Verification items for the finished model (mm, model axes). A direction names the side the tool comes from. Give positions to 0.01 mm unless a question says otherwise; leave off trailing zeros. Write each loop counter-clockwise with the first axis right and the second up, starting at its lowest first coordinate (ties: lowest second). Pieces come first, ordered by that corner, then holes. Notation, with made-up numbers: (-34, 77) -> (-16, 77) arc R18 ccw to (-16, 96) -> close; hole circle Ø9 at (-13.75, 32.5). An arc over 180 degrees is marked (long way). Write item = value, one per line.
from build123d import *

# Parameters (mm, degrees)
F0_R     = 4.5
F0_R_2   = 1.5
F1_DEPTH = 1.5
F2_R     = 4


with BuildPart() as f1:
    # F0 (on Top) → F1 (new body)
    with BuildSketch(Plane.XY):
        with BuildLine():
            ThreePointArc((3.004161691, -5.7955113904), (1.5522577141, -6.3433300134), (0.0118794416, -6.5313863328))
            ThreePointArc((0.0118794416, -6.5313863328), (-1.5361614481, -6.3472667251), (-2.995838309, -5.7998417643))
            Line((-2.995838309, -5.7998417643), (-2.995838309, -10.8488196837))
            ThreePointArc((-2.995838309, -10.8488196837), (-2.764421371, -11.4885696949), (-2.1772781553, -11.8322217287))
            ThreePointArc((-2.1772781553, -11.8322217287), (0.0046169816, -12.0313963001), (2.1863582083, -11.8305428262))
            ThreePointArc((2.1863582083, -11.8305428262), (2.7729908389, -11.4867349425), (3.004161691, -10.8472806897))
            Line((3.004161691, -10.8472806897), (3.004161691, -5.7955113904))
        make_face()
        with BuildLine():
            ThreePointArc((0.0118794416, -6.5313863328), (1.0743113125, -6.9697548816), (1.5146208008, -8.0313838278))
            ThreePointArc((1.5146208008, -8.0313838278), (-1.0450697109, -9.093012774), (0.0118794416, -6.5313863328))
        make_face(mode=Mode.SUBTRACT)
        with BuildLine():
            ThreePointArc((-2.995838309, -5.7998417643), (-1.5361614481, -6.3472667251), (0.0118794416, -6.5313863328))
            ThreePointArc((0.0118794416, -6.5313863328), (1.5522577141, -6.3433300134), (3.004161691, -5.7955113904))
            ThreePointArc((3.004161691, -5.7955113904), (4.5961940777, -4.627591266), (5.7641142021, -3.0355588793))
            ThreePointArc((5.7641142021, -3.0355588793), (6.3133486484, -1.5778863875), (6.5, -0.0313971883))
            ThreePointArc((6.5, -0.0313971883), (6.3144631499, 1.5105350826), (5.768444576, 2.9644411207))
            ThreePointArc((5.768444576, 2.9644411207), (4.5995100863, 4.5614784867), (3.004161691, 5.7327170138))
            ThreePointArc((3.004161691, 5.7327170138), (1.5481312977, 6.2815489928), (0.0033814005, 6.4686019322))
            ThreePointArc((0.0033814005, 6.4686019322), (-1.540289778, 6.2834668165), (-2.995838309, 5.7370473877))
            ThreePointArc((-2.995838309, 5.7370473877), (-4.5961940777, 4.5647968894), (-5.768444576, 2.9644411207))
            ThreePointArc((-5.768444576, 2.9644411207), (-6.4999983071, -0.0360884255), (-5.7641142021, -3.0355588793))
            ThreePointArc((-5.7641142021, -3.0355588793), (-4.592875675, -4.6309072746), (-2.995838309, -5.7998417643))
        make_face()
        with Locations((0, -0.0313971883)):
            Circle(F0_R, mode=Mode.SUBTRACT)
        with BuildLine():
            Line((-10.8158835014, -3.0355588793), (-5.7641142021, -3.0355588793))
            ThreePointArc((-5.7641142021, -3.0355588793), (-6.4999983071, -0.0360884255), (-5.768444576, 2.9644411207))
            Line((-5.768444576, 2.9644411207), (-10.8174224954, 2.9644411207))
            ThreePointArc((-10.8174224954, 2.9644411207), (-11.4571725066, 2.7330241827), (-11.8008245404, 2.145880967))
            ThreePointArc((-11.8008245404, 2.145880967), (-11.9999991118, -0.0360141699), (-11.7991456379, -2.2177553966))
            ThreePointArc((-11.7991456379, -2.2177553966), (-11.4553377541, -2.8043880272), (-10.8158835014, -3.0355588793))
        make_face()
        with Locations((-9.5, -0.0313971883)):
            Circle(F0_R_2, mode=Mode.SUBTRACT)
        with BuildLine():
            ThreePointArc((6.5, -0.0313971883), (6.3133486484, -1.5778863875), (5.7641142021, -3.0355588793))
            Line((5.7641142021, -3.0355588793), (10.8158835014, -3.0355588793))
            ThreePointArc((10.8158835014, -3.0355588793), (11.4553377541, -2.8043880272), (11.7991456379, -2.2177553966))
            ThreePointArc((11.7991456379, -2.2177553966), (11.9999991118, -0.0360141699), (11.8008245404, 2.145880967))
            ThreePointArc((11.8008245404, 2.145880967), (11.4571725066, 2.7330241827), (10.8174224954, 2.9644411207))
            Line((10.8174224954, 2.9644411207), (5.768444576, 2.9644411207))
            ThreePointArc((5.768444576, 2.9644411207), (6.3144631499, 1.5105350826), (6.5, -0.0313971883))
        make_face()
        with Locations((9.5, -0.0313971883)):
            Circle(F0_R_2, mode=Mode.SUBTRACT)
        with BuildLine():
            Line((-2.995838309, 10.7860253071), (-2.995838309, 5.7370473877))
            ThreePointArc((-2.995838309, 5.7370473877), (-1.540289778, 6.2834668165), (0.0033814005, 6.4686019322))
            ThreePointArc((0.0033814005, 6.4686019322), (1.5481312977, 6.2815489928), (3.004161691, 5.7327170138))
            Line((3.004161691, 5.7327170138), (3.004161691, 10.7844863131))
            ThreePointArc((3.004161691, 10.7844863131), (2.7729908389, 11.4239405658), (2.1863582083, 11.7677484496))
            ThreePointArc((2.1863582083, 11.7677484496), (0.0046169816, 11.9686019235), (-2.1772781553, 11.7694273521))
            ThreePointArc((-2.1772781553, 11.7694273521), (-2.764421371, 11.4257753183), (-2.995838309, 10.7860253071))
        make_face()
        with BuildLine():
            ThreePointArc((1.504161691, 7.9686017292), (1.0645459525, 6.907665719), (0.0033814005, 6.4686019322))
            ThreePointArc((0.0033814005, 6.4686019322), (-1.0562225706, 9.0295377395), (1.504161691, 7.9686017292))
        make_face(mode=Mode.SUBTRACT)
    extrude(amount=F1_DEPTH)

    # F2
    f2_edges = [f1.edges().sort_by_distance(p)[0] for p in [
        (-5.764114, -3.035559, 0.75),
        (-2.995838, -5.799842, 0.75),
        (3.004162, 5.732717, 0.75),
        (5.768445, 2.964441, 0.75),
        (5.764114, -3.035559, 0.75),
        (3.004162, -5.795511, 0.75),
        (-2.995838, 5.737047, 0.75),
        (-5.768445, 2.964441, 0.75),
    ]]
    fillet(f2_edges, radius=F2_R)


solid = f1.part
Item 1: Set-up check for faces 4 (the flat face through (3.004, -9, 1)), 5 (the flat face through (5, 0, 0)), 6 (the flat face through (9, 2.964, 1)), 7 (the flat face through (-9, -3.036, 1)), 8 (the flat face through (-9, 2.964, 1)): record each of +Z, -Z, +X, -X, +Y, -Y from which the full face is reachable in a straight line by a thin tool's end or side.
Response values:
face_4 = +Z, -Z, +X, -Y
face_5 = -Z, +X, -X, +Y, -Y
face_6 = +Z, -Z, +X, +Y
face_7 = +Z, -Z, -X, -Y
face_8 = +Z, -Z, -X, +Y
Item 2: Mould release check, pull along Y, two halves, no side actions. Record for faces 1 (the cylindrical face through (-2.76, 11.43, 0.74)), 2 (the cylindrical face through (-3.335, -6.249, 0.76)), 3 (the cylindrical face through (8, 0, 1)): +Y half, -Y half, draft (parallel to the pull), parting line (faces both ways), or undercut.
Response values:
face_1 = +Y half
face_2 = -Y half
face_3 = undercut
Item 3: Sectioned sample at B-B on y = 8.5. Record the cut outline in (x, z), then the cut area to 3 significant figures.
Response values:
outline = (-3, 0) -> (-1.4, 0) -> (-1.4, 1.5) -> (-3, 1.5) -> close; (1.41, 0) -> (3, 0) -> (3, 1.5) -> (1.41, 1.5) -> close
area = 4.79 mm^2
Item 4: Sectioned sample at A-A on x = 9.5. Record the cut outline in (y, z).
Response values:
outline = (-3.04, 0) -> (-1.53, 0) -> (-1.53, 1.5) -> (-3.04, 1.5) -> close; (1.47, 0) -> (2.96, 0) -> (2.96, 1.5) -> (1.47, 1.5) -> close
Item 5: Go/stop test with flat-tipped pins: P1, Ø0.8, axis at x = -9.5, z = 1, coming from the -Y side; P2, Ø0.8, axis at y = 9, z = 0.5, coming from the +X side; P3, Ø8, axis at x = 0, y = -0.03, coming from the +Z side. Record where each tip stops, or that it passes through.
Response values:
P1 = -3.04
P2 = 3
P3 = through
Item 6: Sectioned sample at C-C on z = 0.75. Give the number of separate pieces and of enclosed holes in the cut face, then the cut area to 3 significant figures.
Response values:
separate_pieces = 1
enclosed_holes = 5
area = 179 mm^2
Item 7: Material ranges on line 1 (X direction, y = 0, z = 0.7); line 2 (X direction, y = 1, z = 0.15); line 3 (Y direction, x = 9.5, z = 1.25), recorded low to high.
Response values:
line_1 = -12 to -11, -8 to -4.5, 4.5 to 8, 11 to 12
line_2 = -11.96 to -10.59, -8.41 to -4.38, 4.38 to 8.41, 10.59 to 11.96
line_3 = -3.04 to -1.53, 1.47 to 2.96
